```python
from build123d import *

# Parameters (mm, degrees)
SKETCH1_W           = 105
SKETCH1_H           = 85
BOSS_EXTRUDE1_DEPTH = 3
BOSS_EXTRUDE3_DEPTH = 2.5
BOSS_EXTRUDE2_DEPTH = 2.5
SKETCH4_R           = 4
CUT_EXTRUDE1_DEPTH  = 133.63411713


with BuildPart() as part:
    # Sketch1 → Boss-Extrude1 (new body)
    with BuildSketch(Plane(origin=(0, 0, 0), x_dir=(1, 0, 0), z_dir=(0, 1, 0))):
        with Locations((-6.063023564, 110.481367852)):
            Rectangle(SKETCH1_W, SKETCH1_H)
    extrude(amount=BOSS_EXTRUDE1_DEPTH)

    # Sketch3 → Boss-Extrude3 (add)
    with BuildSketch(Plane.XY.offset(-85.981367852)):
        Polygon((-38, 0), (42, 0), (-23.946113063, -98.352332448), (-52.884605872, -98.352332448), align=None)
    extrude(amount=-BOSS_EXTRUDE3_DEPTH)

    # Sketch2 → Boss-Extrude2 (add)
    with BuildSketch(Plane(origin=(0, 0, -134.981367852), x_dir=(-1, 0, 0), z_dir=(0, 0, -1))):
        Polygon((38, 0), (52.884605872, -98.352332448), (23.946113063, -98.352332448), (-42, 0), align=None)
    extrude(amount=-BOSS_EXTRUDE2_DEPTH)

    # Sketch4 → Cut-Extrude1 (cut, through all)
    with BuildSketch(Plane(origin=(0, 0, -134.981367852), x_dir=(-1, 0, 0), z_dir=(0, 0, -1))):
        with Locations((37.669993982, -88.574319881)):
            Circle(SKETCH4_R)
    extrude(amount=-CUT_EXTRUDE1_DEPTH, mode=Mode.SUBTRACT)


solid = part.part
```
Here's how the part is built. I have some questions about the finished solid (model axes, mm). A direction names the side the tool comes from. Round coordinates to 2 decimals unless told otherwise and drop trailing zeros. Order: outer loops, then holes, each group sorted by start corner. A loop starts at its lowest first (then second) coordinate and runs counter-clockwise, first axis right, second up. Notation, with made-up numbers: M 74.25,49.25 L 132.25,49.25 A14 ccw 132.25,54.25 Z; hole C -38.75,71.25 d1. An arc over 180 degrees is marked long. Answer in a Markdown table with one row per item.
Item 1: I'm going to push flat-ended pins straight in: pin 1 (2 mm diameter, centred on x = -22.5, y = -51.5, fed in from +Z); pin 2 (12 mm diameter, centred on y = -85, z = -89, fed in from +X); pin 3 (1.5 mm diameter, centred on x = -46.5, y = -57, fed in from -Z). Where does each tip first touch, or does it pass through?
A:
| item | result |
|---|---|
| pin 1 | stops at z = -85.98 |
| pin 2 | stops at x = -10.99 |
| pin 3 | stops at z = -134.98 |
Item 2: Imagine slicing it at A-A, the plane y = -3.5. Write out the boundary of the cut face in (x, z), and give its area (3 significant figures).
A:
| item | result |
|---|---|
| outline | M -38.53,-134.98 L 39.65,-134.98 L 39.65,-132.48 L -38.53,-132.48 Z; M -38.53,-88.48 L 39.65,-88.48 L 39.65,-85.98 L -38.53,-85.98 Z |
| area | 391 mm2 |
Item 3: For faces 4 (the face through (-45.34, -48.49, -133.75)), 5 (the face through (-15, -38, -85.981)), 6 (the face through (-17, -38, -134.981)), 7 (the face through (-15, -38, -88.481)), which set-ups out of +Z, -Z, +X, -X, +Y, -Y let a thin tool reach every point of the face, with its end or its side?
A:
| item | result |
|---|---|
| face 4 | +Z, -Z, -X |
| face 5 | +Z, +X, -X, -Y |
| face 6 | -Z, +X, -X, -Y |
| face 7 | +X, -X, -Y |
Item 4: Imagine slicing it at D-D, the plane z = -90.5. Write out the boundary of the cut face in (x, y).
A:
| item | result |
|---|---|
| outline | M -58.56,0 L 46.44,0 L 46.44,3 L -58.56,3 Z |
Item 5: Imagine slicing it at C-C, the plane y = -90.5. Write out the boundary of the cut face in (x, z), and give its area (3 significant figures).
A:
| item | result |
|---|---|
| outline | M -51.7,-134.98 L -41.18,-134.98 L -41.18,-132.48 L -51.7,-132.48 Z; M -51.7,-88.48 L -41.18,-88.48 L -41.18,-85.98 L -51.7,-85.98 Z; M -34.16,-134.98 L -18.68,-134.98 L -18.68,-132.48 L -34.16,-132.48 Z; M -34.16,-88.48 L -18.68,-88.48 L -18.68,-85.98 L -34.16,-85.98 Z |
| area | 130 mm2 |
Item 6: Imagine slicing it at B-B, the plane x = -29. Write out the boundary of the cut face in (y, z), and give its area (3 significant figures).
A:
| item | result |
|---|---|
| outline | M -98.35,-134.98 L 0,-134.98 L 0,-152.98 L 3,-152.98 L 3,-67.98 L 0,-67.98 L 0,-85.98 L -98.35,-85.98 L -98.35,-88.48 L 0,-88.48 L 0,-132.48 L -98.35,-132.48 Z |
| area | 747 mm2 |
Item 7: If I drill on L1, parallel to Z at x = -23, y = -36; L2, parallel to Y at x = -38, z = -104; L3, parallel to X at y = -28.5, z = -134, over which ranges is the centre line in solid material (lowest first)? Write a range as from..to.
A:
| item | result |
|---|---|
| L1 | z = -134.98..-132.48, -88.48..-85.98 |
| L2 | y = 0..3 |
| L3 | x = -42.31..22.89 |
Item 8: Thinking about a two-plate mould opening in Z: for faces 1 (the face through (-7, 1, -152.981)), 2 (the face through (-37.15, -84.61, -133.75)), 3 (the face through (-7, 0, -111)), which applies, +Z half, -Z half, draft (parallel to the pull), parting line (faces both ways), or undercut?
A:
| item | result |
|---|---|
| face 1 | -Z half |
| face 2 | draft |
| face 3 | undercut |
